Model file for the job. Use its own axes, mm. A direction names the side the tool comes from. Coordinates: 2 decimals unless noted, no trailing zeros. Loops run counter-clockwise (first coordinate to the right, second up) from the corner with the lowest first, then second, coordinate; pieces in that order, holes last. Notation, with made-up numbers: (20.25, -36) -> (44.25, -36) arc R29 cw to (44.25, -10) -> close; hole circle Ø9 at (67.5, 74.25). An arc over 180 degrees is marked (long way). Use one line per item in the form item = value.
```python
from build123d import *

# Parameters (mm, degrees)
F0_W     = 15
F0_H     = 150
F1_DEPTH = 10
F2_W     = 10
F2_H     = 5
F3_DEPTH = 15
F4_W     = 5
F4_H     = 90
F5_DEPTH = 10
F6_R     = 5
F7_DEPTH = 5


with BuildPart() as f1:
    # F0 (on Top) → F1 (new body)
    with BuildSketch(Plane.XY):
        with Locations((7.5, -75)):
            Rectangle(F0_W, F0_H)
    extrude(amount=-F1_DEPTH)

    # F2 (on face) → F3 (cut)
    with BuildSketch(Plane.YZ.offset(15)):
        with Locations((-145, -2.5)):
            Rectangle(F2_W, F2_H)
    extrude(amount=-F3_DEPTH, mode=Mode.SUBTRACT)

    # F4 (on face) → F5 (cut)
    with BuildSketch(Plane(origin=(0, 0, -10), x_dir=(1, 0, 0), z_dir=(0, 0, -1))):
        with Locations((12.5, 45)):
            Rectangle(F4_W, F4_H)
    extrude(amount=-F5_DEPTH, mode=Mode.SUBTRACT)

    # F6 (on face) → F7 (join)
    with BuildSketch(Plane(origin=(0, 0, -10), x_dir=(1, 0, 0), z_dir=(0, 0, -1))):
        with Locations((7.5, 105)):
            Circle(F6_R)
    extrude(amount=F7_DEPTH)


solid = f1.part
```
Q1. Band-saw the part on B-B, the plane x = 7.5. Write the cut outline in (y, z).
Result:
outline = (-150, -10) -> (-110, -10) -> (-110, -15) -> (-100, -15) -> (-100, -10) -> (0, -10) -> (0, 0) -> (-140, 0) -> (-140, -5) -> (-150, -5) -> close
Q2. Band-saw the part on C-C, the plane z = -3. Write the cut outline in (x, y).
Result:
outline = (0, -140) -> (15, -140) -> (15, -90) -> (10, -90) -> (10, 0) -> (0, 0) -> close
Q3. Pin check, flat tips, straight feed: pin 1 Ø1.5 at (x, y) = (3, -109.5) entering from -Z; pin 2 Ø1.5 at (x, z) = (12, -4.5) entering from +Y; pin 3 Ø1.5 at (x, z) = (6, -2) entering from -Y. Stop position of each tip, or through.
Result:
pin_1 = -10
pin_2 = -90
pin_3 = -140
Q4. Band-saw the part on A-A, the plane y = -105. Write the cut outline in (x, z).
Result:
outline = (0, -10) -> (2.5, -10) -> (2.5, -15) -> (12.5, -15) -> (12.5, -10) -> (15, -10) -> (15, 0) -> (0, 0) -> close
Q5. Wall check: line 1 along Y through (x, z) = (7.25, -4); line 2 along Z through (x, y) = (3.75, -84.5); line 3 along X through (y, z) = (-30, -2.5). Give the ranges that are in metal, low to high.
Result:
line_1 = -140 to 0
line_2 = -10 to 0
line_3 = 0 to 10
Q6. Band-saw the part on D-D, the plane y = -29. Write the cut outline in (x, z).
Result:
outline = (0, -10) -> (10, -10) -> (10, 0) -> (0, 0) -> close
Q7. Which spindle directions (+Z, -Z, +X, -X, +Y, -Y) get a long thin tool onto all of the face, cutting with end or side? Do faces 1 (the face through (6.42, -100.12, -12.46)), 2 (the face through (12, -90, -5)), 3 (the face through (8, -145, -5)). Say none if no direction does.
Result:
face_1 = -Z
face_2 = +Z, -Z, +X, +Y
face_3 = +Z, +X, -X, -Y
